```python
from build123d import *

# Parameters (mm, degrees)
F1_DEPTH = 25.4


with BuildPart() as f1:
    # F0 (on Front) → F1 (new body)
    with BuildSketch(Plane.XZ):
        Polygon((-34.587627, 39.812567), (-68.589919, 65.314286), (-68.589919, -87.085714), align=None)
        Polygon((81.122858, -46.970297), (-68.589919, -87.085714), (134.610081, -87.085714), (84.258229, -49.321825), (84.258229, -50.733879), (81.122858, -50.733879), align=None)
        Polygon((-34.587627, 39.812567), (-68.589919, -87.085714), (-7.189081, 19.263657), (-31.920042, 37.811878), (-31.920042, 33.991322), (-34.587627, 33.991322), align=None)
        Polygon((-7.189081, 19.263657), (-68.589919, -87.085714), (18.495796, 0), (-4.62309, 17.339164), (-4.62309, 16.45257), (-7.189081, 16.45257), align=None)
        Polygon((18.495796, 0), (-68.589919, -87.085714), (46.225291, -20.797122), (21.687223, -2.39357), (21.687223, -3.414334), (18.495796, -3.414334), align=None)
        Polygon((46.225291, -20.797122), (-68.589919, -87.085714), (81.122858, -46.970297), (48.765291, -22.702122), (46.225291, -22.35774), align=None)
    extrude(amount=F1_DEPTH)


solid = f1.part
```
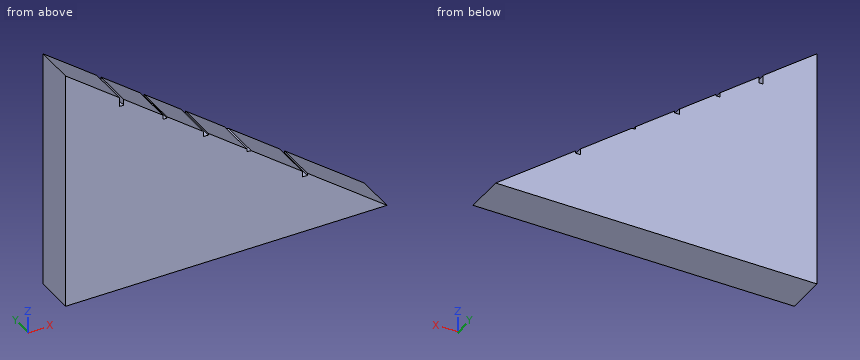
The model under review builds one solid part; all positions refer to its coordinate system, in mm. Round coordinates to 2 decimals unless told otherwise and drop trailing zeros. Loops run counter-clockwise (first coordinate to the right, second up) from the corner with the lowest first, then second, coordinate; pieces in that order, holes last.
1) Wall thickness on line 1 along Z through (x, y) = (-34, -24); line 2 along Z through (x, y) = (-31.5, -5.75); line 3 along X through (y, z) = (-3.5, 11): over which ranges is each line inside the solid? List them lowest first.
Values follow:
line 1: z = -87.09 to 33.99
line 2: z = -87.09 to 37.5
line 3: x = -68.59 to 3.83
2) Consider section B-B on x = 11. State the section outline as (y, z) points, then the cut area to 3 significant figures.
Values follow:
outline: (-25.4, -87.09) - (0, -87.09) - (0, 5.62) - (-25.4, 5.62) - close
area: 2,350 mm2
3) Consider section A-A on y = -15.5. State the section outline as (x, z) points, then the cut area to 3 significant figures.
Values follow:
outline: (-68.59, -87.09) - (134.61, -87.09) - (84.26, -49.32) - (84.26, -50.73) - (81.12, -50.73) - (81.12, -46.97) - (48.77, -22.7) - (46.23, -22.36) - (46.23, -20.8) - (21.69, -2.39) - (21.69, -3.41) - (18.5, -3.41) - (18.5, 0) - (-4.62, 17.34) - (-4.62, 16.45) - (-7.19, 16.45) - (-7.19, 19.26) - (-31.92, 37.81) - (-31.92, 33.99) - (-34.59, 33.99) - (-34.59, 39.81) - (-68.59, 65.31) - close
area: 15,400 mm2
4) Consider section C-C on z = -75. State the section outline as (x, y) points, then the cut area to 3 significant figures.
Values follow:
outline: (-68.59, -25.4) - (118.5, -25.4) - (118.5, 0) - (-68.59, 0) - close
area: 4,750 mm2
5) Clearance check with flat-ended pins moving along their axes: P1, Ø2.5, axis at y = -15.5, z = -2.5, coming from the +X side; P2, Ø0.8, axis at y = -9.5, z = 18.5, coming from the +X side; P3, Ø3, axis at x = 8, y = -10, coming from the +Z side. State where each tip first meets the part, or that it passes through.
Values follow:
P1: stops at x = 23.5
P2: stops at x = -7.19
P3: stops at z = 9
